Design review of the part built by this model. Coordinates are the model's own, in mm. Face numbers are marked on the shaded views. A direction names the side the tool comes from. Give positions to 0.01 mm unless a question says otherwise; leave off trailing zeros. Loops run counter-clockwise (first coordinate to the right, second up) from the corner with the lowest first, then second, coordinate; pieces in that order, holes last. Notation, with made-up numbers: M 7,38 L 51,38 A16 cw 51,50 Z; hole C 71,63.25 d1. An arc over 180 degrees is marked long. Use CSV: the item, a comma, the result in double quotes.
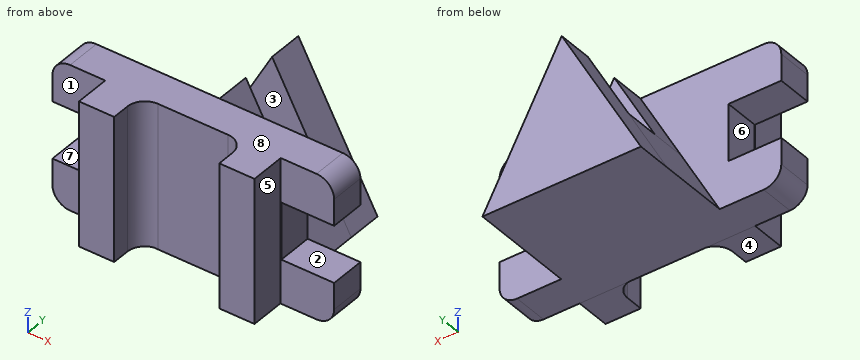
from build123d import *

# Parameters (mm, degrees)
F1_DEPTH  = 25.4
F3_DEPTH  = 25.4
F5_DEPTH  = 25.4
F7_DEPTH  = 25.4
F9_DEPTH  = 25.4
F10_W     = 25.4
F10_H     = 31.75
F11_DEPTH = 25.4
F12_W     = 25.4
F12_H     = 31.75
F12_H_2   = 31.756058
F13_DEPTH = 25.4
F14_W     = 12.7
F14_H     = 19.05
F15_DEPTH = 25.4
F16_W     = 12.7
F16_H     = 19.05
F17_DEPTH = 25.4
F18_W     = 25.4
F18_H     = 25.4
F19_DEPTH = 104.14
F21_DEPTH = 104.14
F23_DEPTH = 104.14


with BuildPart() as f1:
    # F0 (on Front) → F1 (new body)
    with BuildSketch(Plane.XZ):
        Polygon((57.15, 104.473576), (0, 0), (57.15, 0), (57.15, 53.673576), align=None)
        Polygon((57.15, 53.673576), (57.15, 0), (114.3, 0), (57.15, 104.473576), align=None)
    extrude(amount=F1_DEPTH)

    # F2 (on face) → F3 (join)
    with BuildSketch(Plane.XZ.offset(25.4)):
        Polygon((86.422825, 50.961122), (57.15, 50.961122), (27.877175, 50.961122), (0, 0), (114.3, 0), align=None)
    extrude(amount=F3_DEPTH)

    # F4 (on face) → F5 (join)
    with BuildSketch(Plane.XZ.offset(50.8)):
        Polygon((86.422825, 50.961122), (27.877175, 50.961122), (0, 0), (114.3, 0), align=None)
    extrude(amount=F5_DEPTH)

    # F6 (on face) → F7 (join)
    with BuildSketch(Plane.XZ.offset(76.2)):
        Polygon((27.877175, 50.961122), (57.15, 50.961122), (57.15, 104.473576), align=None)
        Polygon((57.15, 104.473576), (57.15, 50.961122), (86.422825, 50.961122), align=None)
    extrude(amount=-F7_DEPTH)

    # F8 (on face) → F9 (join)
    with BuildSketch(Plane.XZ.offset(76.2)):
        Polygon((120.65897, 104.473576), (57.15, 104.473576), (-6.34103, 104.473576), (-6.34103, 0), (120.65897, 0), align=None)
    extrude(amount=F9_DEPTH)

    # F10 (on face) → F11 (join)
    with BuildSketch(Plane.XZ.offset(101.6)):
        with Locations((133.35897, 88.598576)):
            Rectangle(F10_W, F10_H)
        with Locations((133.35897, 15.875)):
            Rectangle(F10_W, F10_H)
    extrude(amount=-F11_DEPTH)

    # F12 (on face) → F13 (join)
    with BuildSketch(Plane.XZ.offset(101.6)):
        with Locations((-19.04103, 15.875)):
            Rectangle(F12_W, F12_H)
        with Locations((-19.04103, 88.595547)):
            Rectangle(F12_W, F12_H_2)
    extrude(amount=-F13_DEPTH)

    # F14 (on face) → F15 (join)
    with BuildSketch(Plane.XZ.offset(101.6)):
        with Locations((-38.09103, 22.225)):
            Rectangle(F14_W, F14_H)
        with BuildLine():
            Line((-31.74103, 0), (-31.74103, 12.7))
            Line((-31.74103, 12.7), (-44.44103, 12.7))
            ThreePointArc((-44.44103, 12.7), (-40.721286, 3.719744), (-31.74103, 0))
        make_face()
        with Locations((-38.09103, 82.242518)):
            Rectangle(F14_W, F14_H)
        with BuildLine():
            Line((-44.44103, 91.767518), (-31.74103, 91.767518))
            Line((-31.74103, 91.767518), (-31.74103, 104.473576))
            ThreePointArc((-31.74103, 104.473576), (-40.723428, 100.75169), (-44.44103, 91.767518))
        make_face()
    extrude(amount=-F15_DEPTH)

    # F16 (on face) → F17 (join)
    with BuildSketch(Plane.XZ.offset(101.6)):
        with Locations((152.40897, 82.248576)):
            Rectangle(F16_W, F16_H)
        with BuildLine():
            Line((146.05897, 104.473576), (146.05897, 91.773576))
            Line((146.05897, 91.773576), (158.75897, 91.773576))
            ThreePointArc((158.75897, 91.773576), (155.039226, 100.753832), (146.05897, 104.473576))
        make_face()
        with Locations((152.40897, 22.225)):
            Rectangle(F16_W, F16_H)
        with BuildLine():
            Line((158.75897, 12.7), (146.05897, 12.7))
            Line((146.05897, 12.7), (146.05897, 0))
            ThreePointArc((146.05897, 0), (155.039226, 3.719744), (158.75897, 12.7))
        make_face()
    extrude(amount=-F17_DEPTH)

    # F18 (on face) → F19 (join)
    with BuildSketch(Plane.XY.offset(104.473576)):
        with Locations((107.532152, -114.3)):
            Rectangle(F18_W, F18_H)
        with Locations((6.33521, -114.3)):
            Rectangle(F18_W, F18_H)
    extrude(amount=-F19_DEPTH)

    # F20 (on face) → F21 (join)
    with BuildSketch(Plane(origin=(0, 0, 0.333576), x_dir=(1, 0, 0), z_dir=(0, 0, -1))):
        with BuildLine():
            Line((19.03521, 114.3), (19.03521, 101.6))
            Line((19.03521, 101.6), (31.73521, 101.6))
            ThreePointArc((31.73521, 101.6), (22.754954, 105.319744), (19.03521, 114.3))
        make_face()
    extrude(amount=-F21_DEPTH)

    # F22 (on face) → F23 (join)
    with BuildSketch(Plane.XY.offset(104.473576)):
        with BuildLine():
            Line((94.832152, -114.3), (94.832152, -101.6))
            Line((94.832152, -101.6), (82.132152, -101.6))
            ThreePointArc((82.132152, -101.6), (91.112408, -105.319744), (94.832152, -114.3))
        make_face()
    extrude(amount=-F23_DEPTH)


solid = f1.part
(1) Machinability: for the marked faces 1, 2, 3 and 4, which of the approach directions +Z, -Z, +X, -X, +Y, -Y give a long, thin tool a straight path to every point of the face, cutting with its end or side? Answer none if there is none.
A:
face 1,"+Z, -Z, -X, -Y"
face 2,"+X, +Y, -Y"
face 3,"+Z, +X, -X"
face 4,"-Z, +X, -X, -Y"
(2) We need section A-A on x = -16. State the section outline as (y, z) points.
A:
outline,"M -101.6,0 L -76.2,0 L -76.2,31.75 L -101.6,31.75 Z; M -101.6,72.72 L -76.2,72.72 L -76.2,104.47 L -101.6,104.47 Z"
(3) The part is to be moulded in two halves that separate along Z. For the marked faces 5, 6, 7 and 8, say which applies: released by +Z, released by -Z, zero draft, split by the parting line, or undercut.
A:
face 5,"zero draft"
face 6,"undercut"
face 7,"undercut"
face 8,"released by +Z"
(4) We need section C-C on z = 75. State the section outline as (x, y) points, then the cut area to 3 significant figures.
A:
outline,"M -44.44,-101.6 L -6.36,-101.6 L -6.36,-127 L 19.04,-127 L 19.04,-114.3 A12.7 cw 31.74,-101.6 L 82.13,-101.6 A12.7 cw 94.83,-114.3 L 94.83,-127 L 120.23,-127 L 120.23,-101.6 L 158.76,-101.6 L 158.76,-76.2 L 73.27,-76.2 L 73.27,-50.8 L 41.03,-50.8 L 41.03,-76.2 L -44.44,-76.2 Z; M 41.03,-25.4 L 73.27,-25.4 L 73.27,0 L 41.03,0 Z"
area,"8,160 mm²"
(5) Wall thickness on line 1 along Y through (x, z) = (59, 84); line 2 along Z through (x, y) = (57, -43.5); line 3 along Y through (x, z) = (132, 14.5): over which ranges is each line inside the solid? List them lowest first. Write a range as [from, to].
A:
line 1,"[-101.6, -50.8], [-25.4, 0]"
line 2,"[0, 50.96]"
line 3,"[-101.6, -76.2]"
(6) We need section D-D on z = 25. State the section outline as (x, y) points, then the cut area to 3 significant figures.
A:
outline,"M -44.44,-101.6 L -6.36,-101.6 L -6.36,-127 L 19.04,-127 L 19.04,-114.3 A12.7 cw 31.74,-101.6 L 82.13,-101.6 A12.7 cw 94.83,-114.3 L 94.83,-127 L 120.23,-127 L 120.23,-101.6 L 158.76,-101.6 L 158.76,-76.2 L 100.62,-76.2 L 100.62,0 L 13.68,0 L 13.68,-76.2 L -44.44,-76.2 Z"
area,"13,100 mm²"
(7) We need section B-B on y = -78.5. State the section outline as (x, z) points, then the cut area to 3 significant figures.
A:
outline,"M -44.44,12.7 A12.7 ccw -31.74,0 L 146.06,0 A12.7 ccw 158.76,12.7 L 158.76,31.75 L 120.66,31.75 L 120.66,72.72 L 158.76,72.72 L 158.76,91.77 A12.7 ccw 146.06,104.47 L -31.74,104.47 A12.7 ccw -44.44,91.77 L -44.44,72.72 L -6.34,72.72 L -6.34,31.75 L -44.44,31.75 Z"
area,"18,000 mm²"
(8) Clearance check with flat-ended pins moving along their axes: P1, Ø1.5, axis at x = 80.5, y = -66.5, coming from the +Z side; P2, Ø12.5, axis at x = 55.5, y = -32.5, coming from the +Z side; P3, Ø7.5, axis at y = -85, z = 53.5, coming from the +X side. State where each tip first meets the part, or that it passes through.
A:
P1,"z = 63.16"
P2,"z = 50.96"
P3,"x = 120.66"
